from build123d import *

# Parameters (mm, degrees)
BOSS_EXTRUDE1_DEPTH = 0.2032


with BuildPart() as part:
    # Sketch1 → Boss-Extrude1 (new body)
    with BuildSketch(Plane(origin=(0, 0, 0), x_dir=(1, 0, 0), z_dir=(0, 1, 0))):
        with BuildLine():
            Line((-1.27, -15.824118459), (-1.27, -34.925))
            Line((-1.27, -34.925), (-2.794, -34.925))
            Line((-2.794, -34.925), (-2.794, -41.275))
            Line((-2.794, -41.275), (-3.556, -41.275))
            Line((-3.556, -41.275), (-3.556, -34.925))
            Line((-3.556, -34.925), (-5.08, -34.925))
            Line((-5.08, -34.925), (-5.08, -15.294253489))
            Line((-5.08, -15.294253489), (-5.08, -15.040253489))
            ThreePointArc((-5.08, -15.040253489), (0, 15.875), (5.08, -15.040253489))
            Line((5.08, -15.040253489), (5.08, -15.294253489))
            Line((5.08, -15.294253489), (5.08, -34.925))
            Line((5.08, -34.925), (3.556, -34.925))
            Line((3.556, -34.925), (3.556, -41.275))
            Line((3.556, -41.275), (2.794, -41.275))
            Line((2.794, -41.275), (2.794, -34.925))
            Line((2.794, -34.925), (1.27, -34.925))
            Line((1.27, -34.925), (1.27, -15.824118459))
            ThreePointArc((1.27, -15.824118459), (0, -15.875), (-1.27, -15.824118459))
        make_face()
    extrude(amount=BOSS_EXTRUDE1_DEPTH)


solid = part.part
Can you work these out from the model? Positions are in its coordinate system, mm. Round coordinates to 2 decimals unless told otherwise and drop trailing zeros. Loops run counter-clockwise (first coordinate to the right, second up) from the corner with the lowest first, then second, coordinate; pieces in that order, holes last. Notation, with made-up numbers: (28.5, 22.25) - (61.5, 22.25) arc R24 cw to (61.5, 39.25) - close; hole circle Ø3 at (44, 69). An arc over 180 degrees is marked (long way). Answer in a Markdown table with one row per item. Add a question column.
Q1. I want a section at C-C on x = 0. List the corners of the cut face in (y, z) for me (3 decimals), and give its area (3 significant figures).
Q2. I need wall thicknesses on L1, parallel to X at y = 0.1, z = 27; L2, parallel to X at y = 0.15, z = 0 (3 decimals); L3, parallel to X at y = 0.15, z = 38.5. Which ranges of each line are inside material? Lowest first, please.
Q3. I want a section at A-A on z = 34. List the corners of the cut face in (x, y) for me, and give its area (3 significant figures).
Q4. I want a section at D-D on z = -11. List the corners of the cut face in (x, y) for me, and give its area (3 significant figures).
Q5. I want a section at B-B on y = 0.1. List the corners of the cut face in (x, z) for me (3 decimals), and give its area (3 significant figures).
A:
| question | item | result |
|---|---|---|
| 1 | outline | (0, -15.875) - (0.203, -15.875) - (0.203, 15.875) - (0, 15.875) - close |
| 1 | area | 6.45 mm^2 |
| 2 | L1 | -5.08 to -1.27, 1.27 to 5.08 |
| 2 | L2 | -15.875 to 15.875 |
| 2 | L3 | -3.56 to -2.79, 2.79 to 3.56 |
| 3 | outline | (-5.08, 0) - (-1.27, 0) - (-1.27, 0.2) - (-5.08, 0.2) - close; (1.27, 0) - (5.08, 0) - (5.08, 0.2) - (1.27, 0.2) - close |
| 3 | area | 1.55 mm^2 |
| 4 | outline | (-11.45, 0) - (11.45, 0) - (11.45, 0.2) - (-11.45, 0.2) - close |
| 4 | area | 4.65 mm^2 |
| 5 | outline | (-5.08, 15.04) arc R15.875 ccw (long way) to (5.08, 15.04) - (5.08, 34.925) - (3.556, 34.925) - (3.556, 41.275) - (2.794, 41.275) - (2.794, 34.925) - (1.27, 34.925) - (1.27, 15.824) arc R15.875 ccw to (-1.27, 15.824) - (-1.27, 34.925) - (-2.794, 34.925) - (-2.794, 41.275) - (-3.556, 41.275) - (-3.556, 34.925) - (-5.08, 34.925) - close |
| 5 | area | 949 mm^2 |
